Geometry: final body of the model. Coordinates: model frame, mm. A direction names the side the tool comes from. Round coordinates to 2 decimals unless told otherwise and drop trailing zeros. Order: outer loops, then holes, each group sorted by start corner. A loop starts at its lowest first (then second) coordinate and runs counter-clockwise, first axis right, second up. Notation, with made-up numbers: M -31,42.5 L -20,42.5 A21 cw -20,78.5 Z; hole C 64,75 d8. An arc over 180 degrees is marked long. Put each result on its own line as item: value. Start each with the question number.
1) Draft query along X for faces 4 (the flat face through (0, 0, 2)), 5 (the flat face through (19, 10, 7)), 6 (the flat face through (0, 9, 3)). Return one class per face: pulls with the +X half, pulls with the -X half, needs draft (parallel to the pull), parting line crosses it, or undercut.
2) Section C-C, the plane x = 0. Return loops of the section in (y, z).
3) Section A-A, the plane z = 10.5. Return loops of the section in (x, y).
4) Section B-B, the plane y = 18.25. Return loops of the section in (x, z), then the cut area to 3 significant figures.
5) First-contact query: P1, Ø3, axis at x = 13, y = 12.5, coming from the +Z side; P2, Ø0.6, axis at x = 5, y = 10.5, coming from the +Z side. Flat tips, straight axial feed; report the tip coordinate or a pass-through.
6) Section D-D, the plane z = 18. Return loops of the section in (x, y) (3 decimals), then the cut area to 3 significant figures.
7) Access query for faces 1 (the flat face through (-9, 4, 14)), 2 (the flat face through (0, 10, 0)), 3 (the flat face through (-16, 10, 8)). Directions: +Z, -Z, +X, -X, +Y, -Y. A direction counts if a zero-diameter tool reaches every point of the face in a straight line with its end or side. Return the directions, or none.
8) Material intervals for probe 1 along X at (y, z) = (11.25, 13.25); probe 2 along Y at (x, z) = (11.5, 2.25); probe 3 along X at (y, z) = (10, 5.75), sorted ascending. Write a range as [from, to].
Autodesk Fusion 360 part; units mm, degrees
sketch "スケッチ1" plane through (0, 0, 0) normal (0, 0, 1) x (1, 0, 0)
  line L0 (-19, 20) -> (19, 20)
  line L1 (19, 20) -> (19, 0)
  line L2 (19, 0) -> (-19, 0)
  line L3 (-19, 0) -> (-19, 20)
  dimension "d1" = 38
  dimension "d2" = 20
extrude "押し出し1" add sketch "スケッチ1" along normal blind 15
sketch "スケッチ2" plane through (0, 0, 0) normal (0, -1, 0) x (1, 0, 0)
  line L0 (-19, 0) -> (19, 0)
  line L1 (19, 0) -> (19, 15)
  line L2 (19, 15) -> (-19, 15)
  line L3 (-19, 15) -> (-19, 0)
  line L4 (-19, 13) -> (19, 13) construction
  arc A0 (-9, 13) -> (9, 13) centre (0, 13) ccw
  line L5 (9, 13) -> (9, 15)
  line L6 (-9, 13) -> (-9, 15)
  dimension "d5" = 2
  dimension "d6" = 18
extrude "押し出し2" cut sketch "スケッチ2" against normal blind 20 contours L2 A0 L5 L6
ref_plane "作業平面1" through (0, 9, 7.5) normal (0, -1, 0) x (1, 0, 0)
sketch "スケッチ3" plane through (0, 9, 6.5) normal (0, -1, 0) x (1, 0, 0)
  line L0 (-16, 8.5) -> (16, 8.5)
  line L1 (16, 8.5) -> (16, -4.5)
  line L2 (16, -4.5) -> (-16, -4.5)
  line L3 (-16, -4.5) -> (-16, 8.5)
  line L4 (-19, 8.5) -> (-9, 8.5)
  arc A0 (-9, 6.5) -> (9, 6.5) centre (0, 6.5) ccw
  line L5 (19, -6.5) -> (19, 8.5)
  dimension "d10" = 32
  dimension "d11" = 11
  dimension "d12" = 3
extrude "押し出し3" cut sketch "スケッチ3" against normal blind 2
sketch "スケッチ4" plane through (0, 0, 15) normal (0, 0, 1) x (-1, 0, 0)
  line L0 (16, -11) -> (9, -11)
  line L1 (9, -11) -> (9, -20)
  line L2 (9, -20) -> (19, -20)
  line L3 (19, -20) -> (19, 0)
  line L4 (19, 0) -> (9, 0)
  line L5 (9, 0) -> (9, -9)
  line L6 (9, -9) -> (16, -9)
  line L7 (16, -9) -> (16, -11)
  line L8 (19, -15.125) -> (-17.5478, -15.125) construction
  line L9 (-19, -20) -> (-9, -20) construction
  line L10 (19, -4.875) -> (-19, -4.875) construction
  line L11 (-19, 0) -> (-19, -20) construction
  circle A0 centre (-15, -15.125) radius 1.5
  circle A1 centre (-15, -4.875) radius 1.5
  circle A2 centre (15, -15.125) radius 1.5
  circle A3 centre (15, -4.875) radius 1.5
  dimension "d15" = 4.875
  dimension "d16" = 10.25
  dimension "d17" = 3
  dimension "d18" = 4
  dimension "d19" = 3
  dimension "d20" = 4
  dimension "d21" = 3
  dimension "d22" = 4
  dimension "d23" = 3
  dimension "d24" = 4
extrude "押し出し4" add sketch "スケッチ4" along normal blind 5 contours A0 | A1 | A2 | A3
Result sheet:
1. face 4: needs draft
1. face 5: pulls with the +X half
1. face 6: undercut
2. outline: M 0,0 L 20,0 L 20,4 L 11,4 L 11,2 L 9,2 L 9,4 L 0,4 Z
3. outline: M -19,0 L -8.65,0 L -8.65,9 L -16,9 L -16,11 L -8.65,11 L -8.65,20 L -19,20 Z; M 8.65,0 L 19,0 L 19,20 L 8.65,20 L 8.65,11 L 16,11 L 16,9 L 8.65,9 Z
4. outline: M -19,0 L 19,0 L 19,15 L 9,15 L 9,13 A9 cw -9,13 L -9,15 L -19,15 Z
4. area: 407 mm2
5. P1: stops at z = 15
5. P2: stops at z = 2
6. outline: C -15,4.875 d3; C -15,15.125 d3; C 15,4.875 d3; C 15,15.125 d3
6. area: 28.3 mm2
7. face 1: +Z, +Y, -Y
7. face 2: -Z, +X, -X, +Y, -Y
7. face 3: +Z
8. probe 1: x = [-19, -9], [9, 19]
8. probe 2: y = [0, 9], [11, 20]
8. probe 3: x = [-19, -16], [16, 19]
